Check sheet for the modelled part. Datum: model origin and axes. Units: mm. Give positions to 0.01 mm unless a question says otherwise; leave off trailing zeros. Order: outer loops, then holes, each group sorted by start corner. A loop starts at its lowest first (then second) coordinate and runs counter-clockwise, first axis right, second up.
Autodesk Inventor part; units mm, degrees
ref_plane "YZ Plane" through (0, 0, 0) normal (1, 0, 0) x (0, 1, 0)
ref_plane "XZ Plane" through (0, 0, 0) normal (0, 1, 0) x (-1, 0, 0)
ref_plane "XY Plane" through (0, 0, 0) normal (0, 0, 1) x (1, 0, 0)
sketch "Sketch1" plane through (0, 0, 0) normal (0, 1, 0) x (-1, 0, 0)
  line L0 (0, 0) -> (253.2063, 0)
  line L1 (253.2063, 0) -> (253.2063, -152.4)
  line L2 (253.2063, -152.4) -> (0, -152.4)
  line L3 (0, -152.4) -> (0, 0)
  line L4 (0, -76.2) -> (56.3563, -76.2)
  circle A0 centre (56.3563, -76.2) radius 4.7625
  dimension "d0" = 152.4
  dimension "d1" = 253.2063
  dimension "d2" = 56.3563
  dimension "d3" = 9.525
extrude "Extrusion1" add sketch "Sketch1" along normal blind 11.9062
sketch "Sketch2" plane through (0, 11.9062, 0) normal (0, 1, 0) x (1, 0, 0)
  line L0 (0, 0) -> (0, 152.4)
  line L1 (0, 76.2) -> (-177.0063, 76.2)
  circle A0 centre (-177.0063, 76.2) radius 7.9375
  dimension "d6" = 177.0062
  dimension "d7" = 15.875
extrude "Extrusion2" cut sketch "Sketch2" against normal blind 11.9062
properties part number "Stage1Wall" material "Wood (Birch)"
1) Section check B-B, the plane x = -179.5. Record the cut outline in (y, z).
Recorded:
outline: (0, -152.4) - (11.91, -152.4) - (11.91, -83.74) - (0, -83.74) - close; (0, -68.66) - (11.91, -68.66) - (11.91, 0) - (0, 0) - close
2) Section check A-A, the plane z = -76.2. Record the cut outline in (x, y).
Recorded:
outline: (-253.21, 0) - (-184.94, 0) - (-184.94, 11.91) - (-253.21, 11.91) - close; (-169.07, 0) - (-61.12, 0) - (-61.12, 11.91) - (-169.07, 11.91) - close; (-51.59, 0) - (0, 0) - (0, 11.91) - (-51.59, 11.91) - close
3) Material ranges on L1, parallel to X at y = 9, z = -76.2; L2, parallel to Z at x = -56.5, y = 2; L3, parallel to Z at x = -180, y = 4.25, recorded low to high.
Recorded:
L1: x = -253.21 to -184.94, -169.07 to -61.12, -51.59 to 0
L2: z = -152.4 to -80.96, -71.44 to 0
L3: z = -152.4 to -83.55, -68.85 to 0
4) Draft check along X on faces 1 (the face through (-253.206, 6, -75)), 2 (the face through (0, 6, -77)), 3 (the face through (-125, 11.906, -75)), 4 (the face through (-182.86, 6.04, -81.56)). Enter one of: +X half, -X half, draft (parallel to the pull), parting line (faces both ways), or undercut.
Recorded:
face 1: -X half
face 2: +X half
face 3: draft
face 4: undercut
